Geometry: final body of the model. Coordinates: model frame, mm. A direction names the side the tool comes from. Give positions to 0.01 mm unless a question says otherwise; leave off trailing zeros. Write each loop counter-clockwise with the first axis right and the second up, starting at its lowest first coordinate (ties: lowest second). Pieces come first, ordered by that corner, then holes.
Q1. Reachability of faces 5 (the face through (37.566, 21.453, 7.042)), 6 (the face through (118, 1, 5)) from +Z, -Z, +X, -X, +Y, -Y: full face, straight path, thin tool, end or side. Return the list, or none.
Q2. Cut plane D-D on x = 60. Return the cut outline in (y, z), plus the area to 3 significant figures.
Q3. Cut plane B-B on z = 6.25. Return the cut outline in (x, y).
Q4. Pin query (flat end, axial travel): pin 1 (6 mm diameter, centred on x = 110, y = 20, fed in from -Z); pin 2 (10 mm diameter, centred on x = 92.5, y = 8.5, fed in from -Z); pin 3 (4 mm diameter, centred on x = 79, y = 18.5, fed in from +Z). Return the tip coordinate at first contact, or that it passes through.
Q5. Cut plane A-A on x = 10. Return the cut outline in (y, z).
Q6. Line query: L1, parallel to Y at x = 110, z = 6.75; L2, parallel to Y at x = 7, z = 8.5; L3, parallel to X at y = 21.5, z = 9. Output: solid intervals per line, ascending.
Q7. Cut plane C-C on y = 40. Return the cut outline in (x, z), plus the area to 3 significant figures.
Q8. Draft query along Y for faces 1 (the face through (59, 30, 10)), 2 (the face through (61.846, 48.951, 7.042)), 3 (the face through (59, 0, 5)), 4 (the face through (42.3, 20.12, 2.03)). Return one class per face: pulls with the +Y half, pulls with the -Y half, needs draft (parallel to the pull), parting line crosses it, or undercut.
```python
from build123d import *

# Parameters (mm, degrees)
SKETCH_1_W          = 120
SKETCH_1_H          = 60
EXTRUDE_1_DEPTH     = 10
SKETCH_2_R          = 3.25
CUT_EXTRUDE_1_DEPTH = 135.536240471
SKETCH_3_R          = 2.25
CUT_EXTRUDE_2_DEPTH = 135.536240471
SKETCH_4_R          = 4
CUT_EXTRUDE_3_DEPTH = 6
FILLET_1_R          = 5


with BuildPart() as part:
    # ｽｹｯﾁ1 → ﾎﾞｽ - 押し出し1 (new body)
    with BuildSketch(Plane.XY):
        with Locations((60, 30)):
            Rectangle(SKETCH_1_W, SKETCH_1_H)
    extrude(amount=EXTRUDE_1_DEPTH)

    # ｽｹｯﾁ2 → ｶｯﾄ - 押し出し1 (cut, through all)
    with BuildSketch(Plane.XY.offset(10)):
        with Locations((10, 40)):
            Circle(SKETCH_2_R)
        with Locations((110, 40)):
            Circle(SKETCH_2_R)
        with Locations(Location((110, 20, 0), (0, 0, 180))):
            Circle(SKETCH_2_R)
        with Locations(Location((10, 20, 0), (0, 0, 180))):
            Circle(SKETCH_2_R)
    extrude(amount=-CUT_EXTRUDE_1_DEPTH, mode=Mode.SUBTRACT)

    # ｽｹｯﾁ3 → ｶｯﾄ - 押し出し2 (cut, through all)
    with BuildSketch(Plane.XY.offset(10)):
        with Locations((60, 52.5)):
            Circle(SKETCH_3_R)
        with Locations((79.485571585, 18.75)):
            Circle(SKETCH_3_R)
        with Locations(Location((40.514428415, 18.75, 0), (0, 0, 180))):
            Circle(SKETCH_3_R)
    extrude(amount=-CUT_EXTRUDE_2_DEPTH, mode=Mode.SUBTRACT)

    # ｽｹｯﾁ4 → ｶｯﾄ - 押し出し3 (cut)
    with BuildSketch(Plane.XY.offset(10)):
        with Locations((60, 52.5)):
            Circle(SKETCH_4_R)
        with Locations((79.485571585, 18.75)):
            Circle(SKETCH_4_R)
        with Locations((40.514428415, 18.75)):
            Circle(SKETCH_4_R)
    extrude(amount=-CUT_EXTRUDE_3_DEPTH, mode=Mode.SUBTRACT)

    # ﾌｨﾚｯﾄ1
    fillet_1_edges = [part.edges().sort_by_distance(p)[0] for p in [
        (0, 60, 5),
        (120, 60, 5),
        (120, 0, 5),
        (0, 0, 5),
    ]]
    fillet(fillet_1_edges, radius=FILLET_1_R)


solid = part.part
```
Data:
1. face 5: +Z
1. face 6: +Z, -Z, +X, -Y
2. outline: (0, 0) - (50.25, 0) - (50.25, 4) - (48.5, 4) - (48.5, 10) - (0, 10) - close; (54.75, 0) - (60, 0) - (60, 10) - (56.5, 10) - (56.5, 4) - (54.75, 4) - close
2. area: 534 mm2
3. outline: (0, 5) arc R5 ccw to (5, 0) - (115, 0) arc R5 ccw to (120, 5) - (120, 55) arc R5 ccw to (115, 60) - (5, 60) arc R5 ccw to (0, 55) - close; hole circle Ø6.5 at (10, 20); hole circle Ø6.5 at (10, 40); hole circle Ø8 at (40.51, 18.75); hole circle Ø8 at (60, 52.5); hole circle Ø8 at (79.49, 18.75); hole circle Ø6.5 at (110, 20); hole circle Ø6.5 at (110, 40)
4. pin 1: passes through
4. pin 2: stops at z = 0
4. pin 3: stops at z = 4
5. outline: (0, 0) - (16.75, 0) - (16.75, 10) - (0, 10) - close; (23.25, 0) - (36.75, 0) - (36.75, 10) - (23.25, 10) - close; (43.25, 0) - (60, 0) - (60, 10) - (43.25, 10) - close
6. L1: y = 0 to 16.75, 23.25 to 36.75, 43.25 to 60
6. L2: y = 0 to 18.75, 21.25 to 38.75, 41.25 to 60
6. L3: x = 0 to 7.12, 12.88 to 37.61, 43.42 to 76.58, 82.39 to 107.12, 112.88 to 120
7. outline: (0, 0) - (6.75, 0) - (6.75, 10) - (0, 10) - close; (13.25, 0) - (106.75, 0) - (106.75, 10) - (13.25, 10) - close; (113.25, 0) - (120, 0) - (120, 10) - (113.25, 10) - close
7. area: 1,070 mm2
8. face 1: needs draft
8. face 2: undercut
8. face 3: pulls with the -Y half
8. face 4: undercut
